from build123d import *

# Parameters (mm, degrees)
SKETCH1_W                   = 140
SKETCH1_H                   = 92
SKETCH1_R                   = 2.5
SKETCH1_R_2                 = 1.5
SKETCH1_W_2                 = 44
SKETCH1_H_2                 = 34
BOSS_EXTRUDE2_DEPTH         = 3
SKETCH3_W                   = 40
SKETCH3_H                   = 35
SKETCH3_R                   = 14.5
BOSS_EXTRUDE3_DEPTH         = 12
SKETCH5_R                   = 2.45
CUT_EXTRUDE1_DEPTH          = 6
SKETCH6_W                   = 9
SKETCH6_H                   = 13
CUT_EXTRUDE3_DEPTH          = 8
SKETCH8_W                   = 29.2
SKETCH8_H                   = 1.5
SKETCH8_W_2                 = 1.5
SKETCH8_H_2                 = 40.2
SKETCH8_W_3                 = 28.2
CUT_EXTRUDE4_DEPTH          = 107.976632963
SKETCH10_R                  = 14.5
CUT_EXTRUDE5_DEPTH          = 107.976632963
SKETCH11_W                  = 19.5
SKETCH11_H                  = 8
CUT_EXTRUDE6_DEPTH          = 108.354552768
SKETCH12_R                  = 2.75
CUT_EXTRUDE7_DEPTH          = 2
SKETCH13_W                  = 5
SKETCH13_H                  = 22
SKETCH13_W_2                = 6
CUT_EXTRUDE8_DEPTH          = 2
ADVANCEDHOLE1_OUTLINE_R     = 1.7
ADVANCEDHOLE1_OUTLINE_R_2   = 1.5
ADVANCEDHOLE1_DEPTH         = 1.45
ADVANCEDHOLE1_DRAFT         = 45
ADVANCEDHOLE1_2_OUTLINE_R   = 1.7
ADVANCEDHOLE1_2_OUTLINE_R_2 = 1.5
ADVANCEDHOLE1_2_DEPTH       = 1.45
ADVANCEDHOLE1_2_DRAFT       = 45
ADVANCEDHOLE1_3_OUTLINE_R   = 1.7
ADVANCEDHOLE1_3_OUTLINE_R_2 = 1.5
ADVANCEDHOLE1_3_DEPTH       = 1.45
ADVANCEDHOLE1_3_DRAFT       = 45
ADVANCEDHOLE1_4_OUTLINE_R   = 1.7
ADVANCEDHOLE1_4_OUTLINE_R_2 = 1.5
ADVANCEDHOLE1_4_DEPTH       = 1.45
ADVANCEDHOLE1_4_DRAFT       = 45


# Read off the part's stored shape, not the designer's step: AdvancedHole1
with BuildPart() as part:
    # Sketch1 → Boss-Extrude2 (new body)
    with BuildSketch(Plane(origin=(0, 0, 0), x_dir=(1, 0, 0), z_dir=(0, 1, 0))):
        with Locations((0, 34)):
            Rectangle(SKETCH1_W, SKETCH1_H)
        with Locations(Location((-5, -2, 0), (0, 0, 270))):
            Circle(SKETCH1_R, mode=Mode.SUBTRACT)
        with Locations(Location((-57.5, 26, 0), (0, 0, 270))):
            Circle(SKETCH1_R_2, mode=Mode.SUBTRACT)
        with Locations(Location((-5.5, 26, 0), (0, 0, 270))):
            Circle(SKETCH1_R_2, mode=Mode.SUBTRACT)
        with Locations(Location((5, -2, 0), (0, 0, 270))):
            Circle(SKETCH1_R, mode=Mode.SUBTRACT)
        with Locations(Location((15, -2, 0), (0, 0, 270))):
            Circle(SKETCH1_R, mode=Mode.SUBTRACT)
        with Locations((-32, 40)):
            Rectangle(SKETCH1_W_2, SKETCH1_H_2, mode=Mode.SUBTRACT)
        with Locations(Location((-57.5, 54, 0), (0, 0, 270))):
            Circle(SKETCH1_R_2, mode=Mode.SUBTRACT)
        with Locations(Location((-5.5, 54, 0), (0, 0, 270))):
            Circle(SKETCH1_R_2, mode=Mode.SUBTRACT)
        with BuildLine():
            ThreePointArc((33.523109919, 48.017542895), (33.981559973, 48.475723098), (34.306815732, 49.036360451))
            ThreePointArc((34.306815732, 49.036360451), (45, 54), (55.693184268, 49.036360451))
            ThreePointArc((55.693184268, 49.036360451), (56.018440027, 48.475723098), (56.476890081, 48.017542895))
            ThreePointArc((56.476890081, 48.017542895), (45, 26), (33.523109919, 48.017542895))
        make_face(mode=Mode.SUBTRACT)
    extrude(amount=BOSS_EXTRUDE2_DEPTH)

    # Sketch3 → Boss-Extrude3 (add)
    with BuildSketch(Plane(origin=(0, 3, 0), x_dir=(1, 0, 0), z_dir=(0, 1, 0))):
        with Locations((45, 40)):
            Rectangle(SKETCH3_W, SKETCH3_H)
        with Locations(Location((45, 40, 0), (0, 0, 270))):
            Circle(SKETCH3_R, mode=Mode.SUBTRACT)
    extrude(amount=BOSS_EXTRUDE3_DEPTH)

    # Sketch5 → Cut-Extrude1 (cut)
    with BuildSketch(Plane(origin=(0, 15, 0), x_dir=(1, 0, 0), z_dir=(0, 1, 0))):
        with Locations((32, 50)):
            Circle(SKETCH5_R)
        with Locations((58, 50)):
            Circle(SKETCH5_R)
        with Locations((58, 30)):
            Circle(SKETCH5_R)
        with Locations((32, 30)):
            Circle(SKETCH5_R)
    extrude(amount=-CUT_EXTRUDE1_DEPTH, mode=Mode.SUBTRACT)

    # Sketch6 → Cut-Extrude3 (cut)
    with BuildSketch(Plane(origin=(0, 15, 0), x_dir=(1, 0, 0), z_dir=(0, 1, 0))):
        with Locations((29.5, 40)):
            Rectangle(SKETCH6_W, SKETCH6_H)
    extrude(amount=-CUT_EXTRUDE3_DEPTH, mode=Mode.SUBTRACT)

    # Sketch8 → Cut-Extrude4 (cut, through all)
    with BuildSketch(Plane(origin=(0, 3, 0), x_dir=(1, 0, 0), z_dir=(0, 1, 0))):
        with Locations((-34.4, 79.25)):
            Rectangle(SKETCH8_W, SKETCH8_H)
        with Locations((34.4, 79.25)):
            Rectangle(SKETCH8_W, SKETCH8_H)
        with Locations((69.25, 34)):
            Rectangle(SKETCH8_W_2, SKETCH8_H_2)
        with Locations((-69.25, 34)):
            Rectangle(SKETCH8_W_2, SKETCH8_H_2)
        with Locations((-34.9, -11.25)):
            Rectangle(SKETCH8_W_3, SKETCH8_H)
        with Locations((34.9, -11.25)):
            Rectangle(SKETCH8_W_3, SKETCH8_H)
    extrude(amount=-CUT_EXTRUDE4_DEPTH, mode=Mode.SUBTRACT)

    # Sketch10 → Cut-Extrude5 (cut, through all)
    with BuildSketch(Plane(origin=(0, 3, 0), x_dir=(1, 0, 0), z_dir=(0, 1, 0))):
        with Locations(Location((45, 40, 0), (0, 0, 136.687767262))):
            Circle(SKETCH10_R)
    extrude(amount=-CUT_EXTRUDE5_DEPTH, mode=Mode.SUBTRACT)

    # Sketch11 → Cut-Extrude6 (cut, through all)
    with BuildSketch(Plane(origin=(0, 15, 0), x_dir=(1, 0, 0), z_dir=(0, 1, 0))):
        with Locations((45, 53.5)):
            Rectangle(SKETCH11_W, SKETCH11_H)
    extrude(amount=-CUT_EXTRUDE6_DEPTH, mode=Mode.SUBTRACT)

    # Sketch12 → Cut-Extrude7 (cut)
    with BuildSketch(Plane(origin=(0, 3, 0), x_dir=(1, 0, 0), z_dir=(0, 1, 0))):
        with Locations(Location((-5, -2, 0), (0, 0, 270))):
            Circle(SKETCH12_R)
        with Locations(Location((5, -2, 0), (0, 0, 270))):
            Circle(SKETCH12_R)
        with Locations(Location((15, -2, 0), (0, 0, 270))):
            Circle(SKETCH12_R)
    extrude(amount=-CUT_EXTRUDE7_DEPTH, mode=Mode.SUBTRACT)

    # Sketch13 → Cut-Extrude8 (cut)
    with BuildSketch(Plane(origin=(0, 3, 0), x_dir=(1, 0, 0), z_dir=(0, 1, 0))):
        with Locations((-58, 40)):
            Rectangle(SKETCH13_W, SKETCH13_H)
        with Locations((-5.5, 40)):
            Rectangle(SKETCH13_W_2, SKETCH13_H)
    extrude(amount=-CUT_EXTRUDE8_DEPTH, mode=Mode.SUBTRACT)


with BuildPart() as advancedhole1_tool:
    # AdvancedHole1 outline → AdvancedHole1 (with draft: the straight prism first)
    with BuildSketch(Plane(origin=(0, 1.45, 0), x_dir=(1, 0, 0), z_dir=(0, 1, 0))):
        with Locations((-57.5, 54)):
            Circle(ADVANCEDHOLE1_OUTLINE_R)
        with Locations((-57.5, 54)):
            Circle(ADVANCEDHOLE1_OUTLINE_R_2, mode=Mode.SUBTRACT)
    extrude(amount=-ADVANCEDHOLE1_DEPTH)
    # AdvancedHole1: the draft: its side faces are tilted about the plane it starts from
    advancedhole1_sides = [advancedhole1_tool.faces().sort_by_distance(p)[0] for p in [
        (-59.2, 0.725, -54),
        (-59, 0.725, -54),
    ]]
    draft(advancedhole1_sides, Plane(origin=(0, 1.45, 0), x_dir=(1, 0, 0), z_dir=(0, 1, 0)), ADVANCEDHOLE1_DRAFT)


with BuildPart() as part_1:
    add(part.part)

    # AdvancedHole1: cut by advancedhole1_tool
    add(advancedhole1_tool.part, mode=Mode.SUBTRACT)


with BuildPart() as advancedhole1_2_tool:
    # AdvancedHole1 2 outline → AdvancedHole1 2 (with draft: the straight prism first)
    with BuildSketch(Plane(origin=(0, 1.45, 0), x_dir=(1, 0, 0), z_dir=(0, 1, 0))):
        with Locations((-57.5, 26)):
            Circle(ADVANCEDHOLE1_2_OUTLINE_R)
        with Locations((-57.5, 26)):
            Circle(ADVANCEDHOLE1_2_OUTLINE_R_2, mode=Mode.SUBTRACT)
    extrude(amount=-ADVANCEDHOLE1_2_DEPTH)
    # AdvancedHole1 2: the draft: its side faces are tilted about the plane it starts from
    advancedhole1_2_sides = [advancedhole1_2_tool.faces().sort_by_distance(p)[0] for p in [
        (-59.2, 0.725, -26),
        (-59, 0.725, -26),
    ]]
    draft(advancedhole1_2_sides, Plane(origin=(0, 1.45, 0), x_dir=(1, 0, 0), z_dir=(0, 1, 0)), ADVANCEDHOLE1_2_DRAFT)


with BuildPart() as part_2:
    add(part_1.part)

    # AdvancedHole1 2: cut by advancedhole1_2_tool
    add(advancedhole1_2_tool.part, mode=Mode.SUBTRACT)


with BuildPart() as advancedhole1_3_tool:
    # AdvancedHole1 3 outline → AdvancedHole1 3 (with draft: the straight prism first)
    with BuildSketch(Plane(origin=(0, 1.45, 0), x_dir=(1, 0, 0), z_dir=(0, 1, 0))):
        with Locations((-5.5, 26)):
            Circle(ADVANCEDHOLE1_3_OUTLINE_R)
        with Locations((-5.5, 26)):
            Circle(ADVANCEDHOLE1_3_OUTLINE_R_2, mode=Mode.SUBTRACT)
    extrude(amount=-ADVANCEDHOLE1_3_DEPTH)
    # AdvancedHole1 3: the draft: its side faces are tilted about the plane it starts from
    advancedhole1_3_sides = [advancedhole1_3_tool.faces().sort_by_distance(p)[0] for p in [
        (-7.2, 0.725, -26),
        (-7, 0.725, -26),
    ]]
    draft(advancedhole1_3_sides, Plane(origin=(0, 1.45, 0), x_dir=(1, 0, 0), z_dir=(0, 1, 0)), ADVANCEDHOLE1_3_DRAFT)


with BuildPart() as part_3:
    add(part_2.part)

    # AdvancedHole1 3: cut by advancedhole1_3_tool
    add(advancedhole1_3_tool.part, mode=Mode.SUBTRACT)


with BuildPart() as advancedhole1_4_tool:
    # AdvancedHole1 4 outline → AdvancedHole1 4 (with draft: the straight prism first)
    with BuildSketch(Plane(origin=(0, 1.45, 0), x_dir=(1, 0, 0), z_dir=(0, 1, 0))):
        with Locations((-5.5, 54)):
            Circle(ADVANCEDHOLE1_4_OUTLINE_R)
        with Locations((-5.5, 54)):
            Circle(ADVANCEDHOLE1_4_OUTLINE_R_2, mode=Mode.SUBTRACT)
    extrude(amount=-ADVANCEDHOLE1_4_DEPTH)
    # AdvancedHole1 4: the draft: its side faces are tilted about the plane it starts from
    advancedhole1_4_sides = [advancedhole1_4_tool.faces().sort_by_distance(p)[0] for p in [
        (-7.2, 0.725, -54),
        (-7, 0.725, -54),
    ]]
    draft(advancedhole1_4_sides, Plane(origin=(0, 1.45, 0), x_dir=(1, 0, 0), z_dir=(0, 1, 0)), ADVANCEDHOLE1_4_DRAFT)


with BuildPart() as part_4:
    add(part_3.part)

    # AdvancedHole1 4: cut by advancedhole1_4_tool
    add(advancedhole1_4_tool.part, mode=Mode.SUBTRACT)


solid = part_4.part
Input: part model. Units: mm. Frame: model coordinates. A direction names the side the tool comes from. Round coordinates to 2 decimals unless told otherwise and drop trailing zeros. Write each loop counter-clockwise with the first axis right and the second up, starting at its lowest first coordinate (ties: lowest second). Pieces come first, ordered by that corner, then holes.
1) Cut plane B-B (z = -40). Return the cut outline in (x, y).
2) Cut plane C-C (y = 13). Return the cut outline in (x, z).
3) Cut plane D-D (z = 2). Return the cut outline in (x, y), then the cut area to 3 significant figures.
4) Ray query, L1, parallel to X at y = 0.6, z = 2; L2, parallel to X at y = 1.8, z = -54; L3, parallel to X at y = 2.3, z = 2. Return the intervals inside material, ascending.
5) Contact query for flat-ended pins moving along their axis: P1, Ø5, axis at x = -57.5, z = -54, coming from the -Y side; P2, Ø6, axis at x = 14.5, z = 2.5, coming from the +Y side; P3, Ø4, axis at y = 11.5, z = -32.5, coming from the -X side; P4, Ø3, axis at x = 47.5, z = -17.5, coming from the -Y side. Output: stop coordinate, or through.
6) Draft query along Z for faces 1 (the flat face through (-68.5, 2, -34)), 2 (the flat face through (0, 1, 12)), 3 (the flat face through (25, 6, -40)), 4 (the flat face through (-60, 1, -80)). Return one class per face: pulls with the +Z half, pulls with the -Z half, needs draft (parallel to the pull), parting line crosses it, or undercut.
7) Cut plane A-A (x = 15). Return the cut outline in (y, z).
8) Reachability of faces 5 (the flat face through (30, 9, -57.5)), 6 (the flat face through (-54, 1, -40)), 7 (the flat face through (-6, 1, -40)), 8 (the flat face through (34, 2, -78.5)) from +Z, -Z, +X, -X, +Y, -Y: full face, straight path, thin tool, end or side. Return the list, or none.
Geometry says:
1. outline: (-68.5, 0) - (-54, 0) - (-54, 3) - (-55.5, 3) - (-55.5, 1) - (-60.5, 1) - (-60.5, 3) - (-68.5, 3) - close; (-10, 0) - (30.5, 0) - (30.5, 7) - (25, 7) - (25, 3) - (-2.5, 3) - (-2.5, 1) - (-8.5, 1) - (-8.5, 3) - (-10, 3) - close; (59.5, 0) - (68.5, 0) - (68.5, 3) - (65, 3) - (65, 15) - (59.5, 15) - close
2. outline: (25, -57.5) - (35.25, -57.5) - (35.25, -50.73) arc R14.5 cw to (34.45, -49.95) arc R2.45 cw (long way) to (32.68, -47.65) arc R14.5 cw to (32.04, -46.5) - (25, -46.5) - close; (25, -33.5) - (32.04, -33.5) arc R14.5 cw to (32.68, -32.35) arc R2.45 cw (long way) to (34.45, -30.05) arc R14.5 cw to (55.55, -30.05) arc R2.45 cw (long way) to (57.32, -32.35) arc R14.5 cw to (57.32, -47.65) arc R2.45 cw (long way) to (55.55, -49.95) arc R14.5 cw to (54.75, -50.73) - (54.75, -57.5) - (65, -57.5) - (65, -22.5) - (25, -22.5) - close
3. outline: (-70, 0) - (-7.5, 0) - (-7.5, 1) - (-7.75, 1) - (-7.75, 3) - (-70, 3) - close; (-2.5, 0) - (2.5, 0) - (2.5, 1) - (2.25, 1) - (2.25, 3) - (-2.25, 3) - (-2.25, 1) - (-2.5, 1) - close; (7.5, 0) - (12.5, 0) - (12.5, 1) - (12.25, 1) - (12.25, 3) - (7.75, 3) - (7.75, 1) - (7.5, 1) - close; (17.5, 0) - (70, 0) - (70, 3) - (17.75, 3) - (17.75, 1) - (17.5, 1) - close
3. area: 372 mm2
4. L1: x = -70 to -7.5, -2.5 to 2.5, 7.5 to 12.5, 17.5 to 70
4. L2: x = -68.5 to -59, -56 to -54, -10 to -7, -4 to 35.25, 54.75 to 68.5
4. L3: x = -70 to -7.75, -2.25 to 2.25, 7.75 to 12.25, 17.75 to 70
5. P1: stops at y = 0.65
5. P2: stops at y = 3
5. P3: stops at x = 25
5. P4: stops at y = 0
6. face 1: undercut
6. face 2: pulls with the +Z half
6. face 3: needs draft
6. face 4: pulls with the -Z half
7. outline: (0, -80) - (3, -80) - (3, -0.75) - (1, -0.75) - (1, -0.5) - (0, -0.5) - close; (0, 4.5) - (1, 4.5) - (1, 4.75) - (3, 4.75) - (3, 12) - (0, 12) - close
8. face 5: -Z, +X, -X, +Y
8. face 6: +Y, -Y
8. face 7: +Y
8. face 8: -Z, +Y, -Y
